Source: three-view drawing plus pictorial views. Frame: mm from the lowest corner of the part. A direction names the side the tool comes from. Give positions to 0.01 mm unless a question says otherwise; leave off trailing zeros. Write each loop counter-clockwise with the first axis right and the second up, starting at its lowest first coordinate (ties: lowest second). Pieces come first, ordered by that corner, then holes. Notation, with made-up numbers: (-2.5, 85.5) -> (36.5, 85.5) arc R29 ccw to (36.5, 115.5) -> close; hole circle Ø5 at (21.5, 58.25). An arc over 180 degrees is marked (long way). Use a Markdown table: item, result. Add a question column.
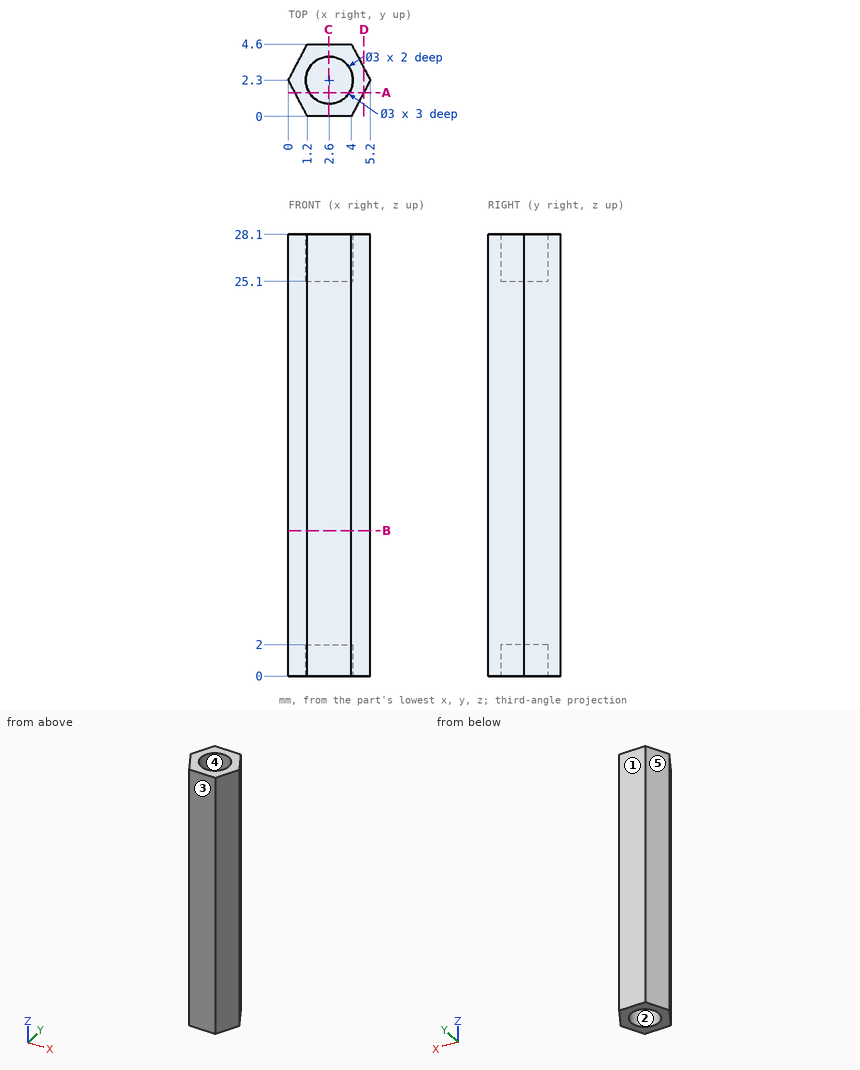
(1) Material intervals for L1, parallel to Z at x = 3.45, y = 1.3; L2, parallel to Y at x = 1.35, z = 1.5; L3, parallel to X at y = 1.85, z = 11 (1 decimal), sorted ascending.
(2) Mould query, pull axis Y, two halves, no side actions, for the marked faces 3, 4 and 5. Classes: +Y half, -Y half, draft (parallel to the pull), parting line (faces both ways), or undercut.
(3) Cut plane B-B on z = 9.25. Return the cut outline in (x, y).
(4) Cut plane C-C on x = 2.55. Return the cut outline in (y, z).
(5) First-contact query: pin 1 Ø1.5 at (x, y) = (2, 2.5) entering from +Z; pin 2 Ø2.5 at (x, y) = (3, 2.5) entering from -Z. Flat tips, straight axial feed; report the tip coordinate or a pass-through.
(6) Access query for the marked faces 1 and 2. Directions: +Z, -Z, +X, -X, +Y, -Y. A direction counts if a zero-diameter tool reaches every point of the face in a straight line with its end or side. Return the directions, or none.
(7) Cut plane D-D on x = 4.8. Return the cut outline in (y, z).
(8) Cut plane A-A on y = 1.5. Return the cut outline in (x, z), then the cut area to 3 significant figures.
Output:
| question | item | result |
|---|---|---|
| 1 | L1 | 2 to 25.1 |
| 1 | L2 | 0 to 1.47, 3.13 to 4.6 |
| 1 | L3 | 0.2 to 5 |
| 2 | face 3 | -Y half |
| 2 | face 4 | undercut |
| 2 | face 5 | +Y half |
| 3 | outline | (0, 2.3) -> (1.2, 0) -> (4, 0) -> (5.2, 2.3) -> (4, 4.6) -> (1.2, 4.6) -> close |
| 4 | outline | (0, 0) -> (0.8, 0) -> (0.8, 2) -> (3.8, 2) -> (3.8, 0) -> (4.6, 0) -> (4.6, 28.1) -> (3.8, 28.1) -> (3.8, 25.1) -> (0.8, 25.1) -> (0.8, 28.1) -> (0, 28.1) -> close |
| 5 | pin 1 | z = 25.1 |
| 5 | pin 2 | z = 0 |
| 6 | face 1 | +Z, -Z, +X, -X, +Y |
| 6 | face 2 | -Z |
| 7 | outline | (1.53, 0) -> (3.07, 0) -> (3.07, 28.1) -> (1.53, 28.1) -> close |
| 8 | outline | (0.42, 0) -> (1.33, 0) -> (1.33, 2) -> (3.87, 2) -> (3.87, 0) -> (4.78, 0) -> (4.78, 28.1) -> (3.87, 28.1) -> (3.87, 25.1) -> (1.33, 25.1) -> (1.33, 28.1) -> (0.42, 28.1) -> close |
| 8 | area | 110 mm^2 |
